from build123d import *

# Parameters (mm, degrees)
SKETCH1_W                   = 40
SKETCH1_H                   = 20
BOSS_EXTRUDE1_DEPTH         = 3
SKETCH2_W                   = 3
SKETCH2_H                   = 20
BOSS_EXTRUDE2_DEPTH         = 15
CUT_EXTRUDE1_REACH          = 46.989
SKETCH4_R                   = 3
FILLET1_RADIUS              = 10
FILLET1_LENGTH              = 3
CUT_EXTRUDE3_REACH          = 46.989
FILLET1_OF_MIRROR1_2_RADIUS = 10
FILLET1_OF_MIRROR1_2_LENGTH = 3
CUT_EXTRUDE2_REACH          = 30.21
SKETCH6_R                   = 1.5


with BuildPart() as part:
    # Sketch1 → Boss-Extrude1 (new body)
    with BuildSketch(Plane(origin=(0, 0, 0), x_dir=(1, 0, 0), z_dir=(0, 1, 0))):
        Rectangle(SKETCH1_W, SKETCH1_H)
    extrude(amount=BOSS_EXTRUDE1_DEPTH)

    # Sketch2 → Boss-Extrude2 (add)
    with BuildSketch(Plane(origin=(0, 3, 0), x_dir=(1, 0, 0), z_dir=(0, 1, 0))):
        with Locations((-18.5, 0)):
            Rectangle(SKETCH2_W, SKETCH2_H)
    boss_extrude2 = extrude(amount=BOSS_EXTRUDE2_DEPTH)

    # Sketch4 → Cut-Extrude1 (cut, up to next)
    with BuildSketch(Plane.ZY.offset(20), mode=Mode.PRIVATE) as cut_extrude1_sk1:
        with Locations((0, 10)):
            Circle(SKETCH4_R)
    cut_extrude1_tool1 = extrude(cut_extrude1_sk1.sketch, amount=-CUT_EXTRUDE1_REACH, mode=Mode.PRIVATE) & part.part
    cut_extrude1 = cut_extrude1_tool1.solids().sort_by_distance((-20, 10, 0))[0]
    add(cut_extrude1, mode=Mode.SUBTRACT)

    # Fillet1: full round fillet: the end face becomes a half cylinder, R = half its width
    fillet1_face = Plane((-18.5, 18, 0), x_dir=(1, 0, 0), z_dir=(0, 1, 0))  # on the end face: x along it, z out of the body
    fillet1_slab = fillet1_face.offset(-FILLET1_RADIUS / 2) * Box(FILLET1_LENGTH, 2 * FILLET1_RADIUS, FILLET1_RADIUS, mode=Mode.PRIVATE)  # the body's end, R deep
    fillet1_round = Plane((-18.5, 8, 0), x_dir=(0, 1, 0), z_dir=(1, 0, 0)) * Cylinder(FILLET1_RADIUS, FILLET1_LENGTH, mode=Mode.PRIVATE)  # its axis R under the face
    add(fillet1_slab - fillet1_round, mode=Mode.SUBTRACT)

    # Sketch8 → Cut-Extrude3 (cut, up to next)
    with BuildSketch(Plane.ZY.offset(20), mode=Mode.PRIVATE) as cut_extrude3_sk1:
        Polygon((0, 7), (5, 20), (-5, 20), align=None)
    cut_extrude3_tool1 = extrude(cut_extrude3_sk1.sketch, amount=-CUT_EXTRUDE3_REACH, mode=Mode.PRIVATE) & part.part
    cut_extrude3 = cut_extrude3_tool1.solids().sort_by_distance((-20, 15.666667, 0))[0]
    add(cut_extrude3, mode=Mode.SUBTRACT)

    # Mirror1: Boss-Extrude2, Cut-Extrude1, Cut-Extrude3 across plane
    add(boss_extrude2.mirror(Plane(origin=(0, 0, 0), x_dir=(0, 0, 1), z_dir=(1, 0, 0))))
    add(cut_extrude1.mirror(Plane(origin=(0, 0, 0), x_dir=(0, 0, 1), z_dir=(1, 0, 0))), mode=Mode.SUBTRACT)
    add(cut_extrude3.mirror(Plane(origin=(0, 0, 0), x_dir=(0, 0, 1), z_dir=(1, 0, 0))), mode=Mode.SUBTRACT)

    # Fillet1 of Mirror1 2: full round fillet: the end face becomes a half cylinder, R = half its width
    fillet1_of_mirror1_2_face = Plane((18.5, 18, 0), x_dir=(-1, 0, 0), z_dir=(0, 1, 0))  # on the end face: x along it, z out of the body
    fillet1_of_mirror1_2_slab = fillet1_of_mirror1_2_face.offset(-FILLET1_OF_MIRROR1_2_RADIUS / 2) * Box(FILLET1_OF_MIRROR1_2_LENGTH, 2 * FILLET1_OF_MIRROR1_2_RADIUS, FILLET1_OF_MIRROR1_2_RADIUS, mode=Mode.PRIVATE)  # the body's end, R deep
    fillet1_of_mirror1_2_round = Plane((18.5, 8, 0), x_dir=(0, 1, 0), z_dir=(-1, 0, 0)) * Cylinder(FILLET1_OF_MIRROR1_2_RADIUS, FILLET1_OF_MIRROR1_2_LENGTH, mode=Mode.PRIVATE)  # its axis R under the face
    add(fillet1_of_mirror1_2_slab - fillet1_of_mirror1_2_round, mode=Mode.SUBTRACT)

    # Sketch6 → Cut-Extrude2 (cut, up to next)
    with BuildSketch(Plane.XZ, mode=Mode.PRIVATE) as cut_extrude2_sk1:
        with Locations(Location((0, 0, 0), (0, 0, 270))):
            Circle(SKETCH6_R)
    cut_extrude2_tool1 = extrude(cut_extrude2_sk1.sketch, amount=-CUT_EXTRUDE2_REACH, mode=Mode.PRIVATE) & part.part
    add(cut_extrude2_tool1.solids().sort_by_distance((0, 0, 0))[0], mode=Mode.SUBTRACT)


solid = part.part
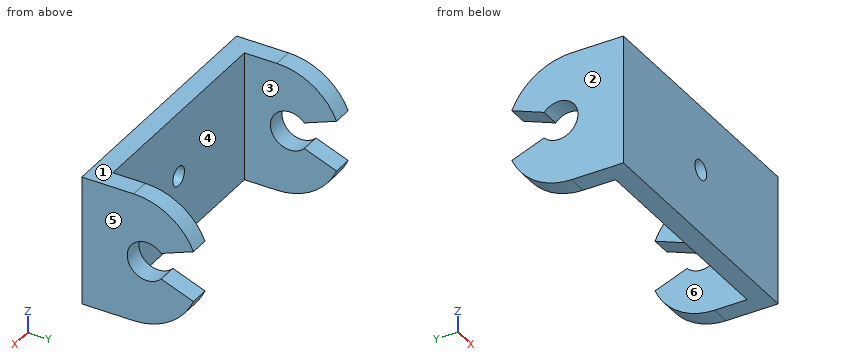
Could you check a few things on this model? Use its own coordinates, in mm. Face numbers are marked on the shaded views. A direction names the side the tool comes from. Give positions to 0.01 mm unless a question says otherwise; leave off trailing zeros. Order: outer loops, then holes, each group sorted by start corner. A loop starts at its lowest first (then second) coordinate and runs counter-clockwise, first axis right, second up. Notation, with made-up numbers: (47.5, 22) -> (80.5, 22) arc R22 cw to (80.5, 46) -> close; hole circle Ø3 at (57, 77). An arc over 180 degrees is marked (long way). Return JSON: item names as keys, results as strings.
1. Imagine slicing it at B-B on z = 0. List the corners of the cut face in (x, y) for me.
Answer list:
{"outline": "(-20, 0) -> (-1.5, 0) -> (-1.5, 3) -> (-17, 3) -> (-17, 7) -> (-20, 7) -> close; (1.5, 0) -> (20, 0) -> (20, 7) -> (17, 7) -> (17, 3) -> (1.5, 3) -> close"}
2. Thinking about a two-plate mould opening in X: for the marked faces 1, 2, 3 and 4, which applies, pulls with the +X half, pulls with the -X half, needs draft (parallel to the pull), parting line crosses it, or undercut?
Answer list:
{"face 1": "needs draft", "face 2": "pulls with the -X half", "face 3": "undercut", "face 4": "undercut"}
3. Imagine slicing it at A-A on y = 4.75. List the corners of the cut face in (x, z) for me, then the cut area to 3 significant figures.
Answer list:
{"outline": "(-20, -10) -> (-17, -10) -> (-17, 10) -> (-20, 10) -> close; (17, -10) -> (20, -10) -> (20, 10) -> (17, 10) -> close", "area": "120 mm2"}
4. Imagine slicing it at D-D on y = 10. List the corners of the cut face in (x, z) for me, then the cut area to 3 significant figures.
Answer list:
{"outline": "(-20, -9.8) -> (-17, -9.8) -> (-17, -3) -> (-20, -3) -> close; (-20, 3) -> (-17, 3) -> (-17, 9.8) -> (-20, 9.8) -> close; (17, -9.8) -> (20, -9.8) -> (20, -3) -> (17, -3) -> close; (17, 3) -> (20, 3) -> (20, 9.8) -> (17, 9.8) -> close", "area": "81.6 mm2"}
5. On a 3-axis mill with a long thin cutter (end or side, diameter ignored), from which of +Z, -Z, +X, -X, +Y, -Y can I reach the whole of each face in a straight line? I mean the marked faces 5 and 6. Say none if no direction works.
Answer list:
{"face 5": "+Z, -Z, +X, +Y, -Y", "face 6": "+Z, -Z, +Y"}
6. I need wall thicknesses on line 1 (X direction, y = 1, z = 0); line 2 (X direction, y = 8.25, z = 6.5); line 3 (Y direction, x = -19.3, z = 0). Which ranges of each line are inside material? Lowest first, please. Write a range as from..to.
Answer list:
{"line 1": "x = -20..-1.5, 1.5..20", "line 2": "x = -20..-17, 17..20", "line 3": "y = 0..7"}
7. Imagine slicing it at C-C on x = 0. List the corners of the cut face in (y, z) for me.
Answer list:
{"outline": "(0, -10) -> (3, -10) -> (3, -1.5) -> (0, -1.5) -> close; (0, 1.5) -> (3, 1.5) -> (3, 10) -> (0, 10) -> close"}
8. For pin 1 Ø1.5 at (x, z) = (4, 3.5) entering from +Y; pin 2 Ø3 at (x, z) = (-7.5, -4) entering from -Y; pin 3 Ø10 at (x, y) = (13, 11.5) entering from +Z, each with a flat end and sliding along its axis, tell me the tip position at first contact or that it passes through.
Answer list:
{"pin 1": "stops at y = 3", "pin 2": "stops at y = 0", "pin 3": "stops at z = 9.99"}
